Design review of the part built by this model. Coordinates are the model's own, in mm. A direction names the side the tool comes from. Coordinates: 2 decimals unless noted, no trailing zeros. Loops run counter-clockwise (first coordinate to the right, second up) from the corner with the lowest first, then second, coordinate; pieces in that order, holes last. Notation, with made-up numbers: (30, 64) -> (49, 64) arc R15 cw to (49, 69) -> close; hole circle Ø3 at (77, 55). An arc over 180 degrees is marked (long way). One line per item, written item: value. Start each with the question number.
1. Machinability: for faces 4 (the flat face through (2, 0, -2)), 5 (the flat face through (-3, 15, 1)), which of the approach directions +Z, -Z, +X, -X, +Y, -Y give a long, thin tool a straight path to every point of the face, cutting with its end or side? Answer none if there is none.
2. For probe 1 along Z at (x, y) = (0, 0.95); probe 2 along Z at (x, y) = (0, 14); probe 3 along Y at (x, z) = (-0.5, 1.25), list the stretches that pass through material, from the lowest coordinate up.
3. Draft analysis for pull direction Z (two halves, no side actions). For faces 1 (the flat face through (-1, 20, -1)), 2 (the cylindrical face through (0.867, 7.402, 3.905)), 3 (the cylindrical face through (0, 9, -1)), state which applies: pulls with the +Z half, pulls with the -Z half, needs draft (parallel to the pull), parting line crosses it, or undercut.
4. Add section C-C on y = -1. Write out the cut boundary in (x, z), plus the area to 3 significant figures.
5. Add section D-D on y = 6.75. Write out the cut boundary in (x, z).
6. Insertion check: pin 1 (4 mm diameter, centred on y = 16.5, z = -1.5, fed in from +X); pin 2 (2 mm diameter, centred on x = -1.5, y = 1.5, fed in from -Z). Each pin has a flat end and moves straight along its axis. Give the tip position at first contact, or say it passes through.
Autodesk Inventor part; units mm, degrees
ref_plane "YZ Plane" through (0, 0, 0) normal (1, 0, 0) x (0, 1, 0)
ref_plane "XZ Plane" through (0, 0, 0) normal (0, 1, 0) x (-1, 0, 0)
ref_plane "XY Plane" through (0, 0, 0) normal (0, 0, 1) x (1, 0, 0)
sketch "Sketch1" plane through (0, 0, 0) normal (0, 0, 1) x (1, 0, 0)
  line L0 (-3, 20) -> (-3, 15)
  line L1 (-3, 15) -> (-4, 15)
  line L2 (-4, 15) -> (-4, 0)
  line L3 (-1.3, 2) -> (-1.3, -3)
  line L4 (-1.3, -3) -> (-1, -3)
  line L5 (-1, -3) -> (-1, 20)
  line L6 (-1, 20) -> (-3, 20)
  line L7 (-1.3, 2) -> (-2.1, 2)
  line L8 (-2.1, 2) -> (-2.1, 0)
  line L9 (-2.1, 0) -> (-4, 0)
  line L10 (0, -7.6) -> (0, 24.6)
  point P0 (0, 0)
  dimension "d0" = 1
  dimension "d1" = 1.3
  dimension "d3" = 15
  dimension "d4" = 2
  dimension "d5" = 5
  dimension "d6" = 4
  dimension "d7" = 0.8
  dimension "d8" = 2
  dimension "d9" = 5
revolve "Revolution1" add sketch "Sketch1" angle 360 about axis through (0, -10, 0) along (0, 1, 0)
chamfer "Chamfer1" distance 0.5 angle 45 3 edges at (4, 15, 0) (3, 20, 0) (4, 0, 0)
chamfer "Chamfer2" distance 0.1 angle 45 4 edges at (2.1, 0, 0) (1.3, -3, 0) (1, -3, 0) (1, 20, 0)
properties part number "EPR Capillary Glue Ferrule"
Worked answers:
1. face 4: -Y
1. face 5: +Y
2. probe 1: z = -4 to -2.1, -1.3 to -1, 1 to 1.3, 2.1 to 4
2. probe 2: z = -4 to -1, 1 to 4
2. probe 3: y = 2 to 20
3. face 1: needs draft
3. face 2: parting line crosses it
3. face 3: undercut
4. outline: circle Ø2.6 at (0, 0); hole circle Ø2 at (0, 0)
4. area: 2.17 mm²
5. outline: circle Ø8 at (0, 0); hole circle Ø2 at (0, 0)
6. pin 1: stops at x = 3.81
6. pin 2: stops at z = -3.97
